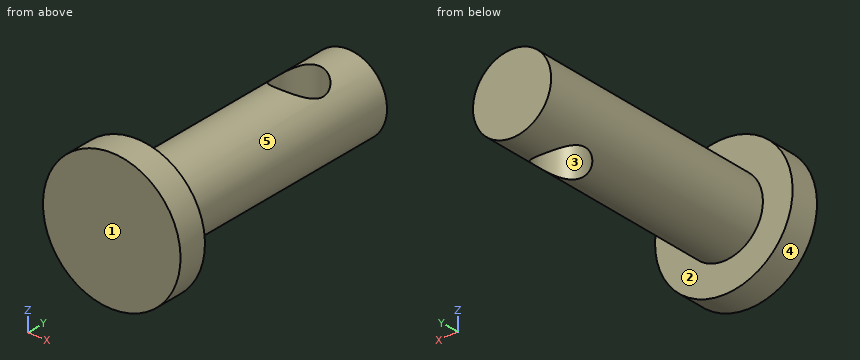
```python
from build123d import *

# Parameters (mm, degrees)
SKETCH1_R               = 3.95
BOSS_EXTRUDE1_DEPTH     = 26
CUT_EXTRUDE1_DEPTH      = 27.59332623
CUT_EXTRUDE1_DEPTH_BACK = 27.59332623
SKETCH2_R               = 2.45
SKETCH3_R               = 6.95
BOSS_EXTRUDE2_DEPTH     = 3


with BuildPart() as part:
    # Sketch1 → Boss-Extrude1 (new body)
    with BuildSketch(Plane(origin=(0, 0, 0), x_dir=(1, 0, 0), z_dir=(0, 1, 0))):
        with Locations(Location((0, 0, 0), (0, 0, 270))):
            Circle(SKETCH1_R)
    extrude(amount=BOSS_EXTRUDE1_DEPTH)

    # Sketch2 → Cut-Extrude1 (cut, two sides: drawn at the far end of the back side and taken through both)
    with BuildSketch(Plane.XY.offset(-CUT_EXTRUDE1_DEPTH_BACK)):
        with Locations((0, 20)):
            Circle(SKETCH2_R)
    extrude(amount=CUT_EXTRUDE1_DEPTH + CUT_EXTRUDE1_DEPTH_BACK, mode=Mode.SUBTRACT)

    # Sketch3 → Boss-Extrude2 (add)
    with BuildSketch(Plane.XZ):
        with Locations(Location((0, 0, 0), (0, 0, 270))):
            Circle(SKETCH3_R)
    extrude(amount=BOSS_EXTRUDE2_DEPTH)


solid = part.part
```
Geometry check sheet. Reference: the model listing, model coordinates, mm. Face numbers are marked on the shaded views. A direction names the side the tool comes from. Give positions to 0.01 mm unless a question says otherwise; leave off trailing zeros. Write each loop counter-clockwise with the first axis right and the second up, starting at its lowest first coordinate (ties: lowest second). Pieces come first, ordered by that corner, then holes.
1) Material ranges on L1, parallel to Y at x = 0, z = -1.75; L2, parallel to Y at x = -3, z = -5.75; L3, parallel to Y at x = 1.5, z = -1.25, recorded low to high.
2) Access from +Z, -Z, +X, -X, +Y, -Y to the whole of each face (thin tool, end or side, straight path). Record for the marked faces 4 and 5.
3) Release check for a two-part mould opening along Y. For the marked faces 1, 2 and 3 record: pulls with the +Y half, pulls with the -Y half, needs draft (parallel to the pull), parting line crosses it, or undercut.
4) Section check A-A, the plane x = 0. Record the boundary of the cut face in (y, z), and give its area (3 significant figures).
5) Section check B-B, the plane z = 0. Record the boundary of the cut face in (x, y), and give its area (3 significant figures).
6) Gauge pin test, flat ends, axial feed: pin 1 (2 mm diameter, centred on y = 20, z = -2.5, fed in from -X); pin 2 (1.5 mm diameter, centred on x = 1, y = 16.5, fed in from -Z); pin 3 (1.5 mm diameter, centred on x = 3, y = 0, fed in from +Z). Record the tip position at first contact, or that the pin passes through.
7) Section check C-C, the plane x = -3.5. Record the boundary of the cut face in (y, z).
8) Section check D-D, the plane x = 2. Record the boundary of the cut face in (y, z), and give its area (3 significant figures).
Computed:
1. L1: y = -3 to 17.55, 22.45 to 26
1. L2: y = -3 to 0
1. L3: y = -3 to 18.06, 21.94 to 26
2. face 4: +Y, -Y
2. face 5: +Y
3. face 1: pulls with the -Y half
3. face 2: pulls with the +Y half
3. face 3: undercut
4. outline: (-3, -6.95) - (0, -6.95) - (0, -3.95) - (17.55, -3.95) - (17.55, 3.95) - (0, 3.95) - (0, 6.95) - (-3, 6.95) - close; (22.45, -3.95) - (26, -3.95) - (26, 3.95) - (22.45, 3.95) - close
4. area: 208 mm2
5. outline: (-6.95, -3) - (6.95, -3) - (6.95, 0) - (3.95, 0) - (3.95, 26) - (-3.95, 26) - (-3.95, 0) - (-6.95, 0) - close; hole circle Ø4.9 at (0, 20)
5. area: 228 mm2
6. pin 1: stops at x = -3.65
6. pin 2: stops at z = -3.94
6. pin 3: stops at z = 6.58
7. outline: (-3, -6) - (0, -6) - (0, -1.83) - (26, -1.83) - (26, 1.83) - (0, 1.83) - (0, 6) - (-3, 6) - close
8. outline: (-3, -6.66) - (0, -6.66) - (0, -3.41) - (18.58, -3.41) - (18.58, 3.41) - (0, 3.41) - (0, 6.66) - (-3, 6.66) - close; (21.42, -3.41) - (26, -3.41) - (26, 3.41) - (21.42, 3.41) - close
8. area: 198 mm2
